Input: part model. Units: mm. Frame: model coordinates. A direction names the side the tool comes from. Give positions to 0.01 mm unless a question says otherwise; leave off trailing zeros. Loops run counter-clockwise (first coordinate to the right, second up) from the corner with the lowest first, then second, coordinate; pieces in that order, holes last. Notation, with made-up numbers: M 27,61.5 L 75,61.5 A10 cw 75,71.5 Z; hole C 10,-21 d10. An arc over 180 degrees is marked long. Use a Markdown table: item, result. Add a question column.
from build123d import *

# Parameters (mm, degrees)
CROQUIS1_W              = 45
CROQUIS1_H              = 20
SALIENTE_EXTRUIR1_DEPTH = 10
CROQUIS2_W              = 40.2
CROQUIS2_H              = 16.2
CORTAR_EXTRUIR1_DEPTH   = 8
CROQUIS3_W              = 14
CROQUIS3_H              = 7
CORTAR_EXTRUIR2_DEPTH   = 8
CROQUIS4_W              = 20
CROQUIS4_H              = 8
CORTAR_EXTRUIR3_DEPTH   = 8


with BuildPart() as part:
    # Croquis1 → Saliente-Extruir1 (new body)
    with BuildSketch(Plane(origin=(0, 0, 0), x_dir=(1, 0, 0), z_dir=(0, 1, 0))):
        Rectangle(CROQUIS1_W, CROQUIS1_H)
    extrude(amount=SALIENTE_EXTRUIR1_DEPTH)

    # Croquis2 → Cortar-Extruir1 (cut)
    with BuildSketch(Plane(origin=(0, 10, 0), x_dir=(1, 0, 0), z_dir=(0, 1, 0))):
        Rectangle(CROQUIS2_W, CROQUIS2_H)
    extrude(amount=-CORTAR_EXTRUIR1_DEPTH, mode=Mode.SUBTRACT)

    # Croquis3 → Cortar-Extruir2 (cut)
    with BuildSketch(Plane(origin=(22.5, 0, 0), x_dir=(0, 0, -1), z_dir=(1, 0, 0))):
        with Locations((0, 6.5)):
            Rectangle(CROQUIS3_W, CROQUIS3_H)
    extrude(amount=-CORTAR_EXTRUIR2_DEPTH, mode=Mode.SUBTRACT)

    # Croquis4 → Cortar-Extruir3 (cut)
    with BuildSketch(Plane.XY.offset(10)):
        with Locations((-10.1, 6)):
            Rectangle(CROQUIS4_W, CROQUIS4_H)
    extrude(amount=-CORTAR_EXTRUIR3_DEPTH, mode=Mode.SUBTRACT)


solid = part.part
1) Reachability of faces 5 (the flat face through (21, 6, 7)), 6 (the flat face through (-22.5, 5, 0)), 7 (the flat face through (0, 6, -8.1)), 8 (the flat face through (-0.1, 6, 9)) from +Z, -Z, +X, -X, +Y, -Y: full face, straight path, thin tool, end or side. Return the list, or none.
2) Ray query, line 1 (Z direction, x = 18, y = 6.5); line 2 (X direction, y = 2.5, z = -0.5); line 3 (X direction, y = 9.75, z = 2.5). Return the intervals inside material, ascending. Write a range as [from, to].
3) Pull-direction query (X, two-part tool) for faces 1 (the flat face through (22.5, 2.7, 0.1)), 2 (the flat face through (0, 2, 1)), 3 (the flat face through (10, 6, 8.1)), 4 (the flat face through (21, 6, -7)); classes: pulls with the +X half, pulls with the -X half, needs draft (parallel to the pull), parting line crosses it, or undercut.
4) Contact query for flat-ended pins moving along their axis: P1, Ø5, axis at x = -1, z = -2.5, coming from the +Y side; P2, Ø1.9, axis at x = 21.5, z = -3, coming from the +Y side; P3, Ø2.5, axis at y = 5, z = 2, coming from the +X side. Output: stop coordinate, or through.
5) Section query B-B, the plane z = -3. Return the cut outline in (x, y).
6) Section query C-C, the plane x = 17.5. Return the cut outline in (y, z), and give its area (3 significant figures).
7) Section query A-A, the plane y = 5.5. Return the cut outline in (x, z).
Entries:
| question | item | result |
|---|---|---|
| 1 | face 5 | +X, +Y |
| 1 | face 6 | +Z, -Z, -X, +Y, -Y |
| 1 | face 7 | +Y |
| 1 | face 8 | +Z, +Y |
| 2 | line 1 | z = [-10, -8.1], [8.1, 10] |
| 2 | line 2 | x = [-22.5, -20.1], [20.1, 22.5] |
| 2 | line 3 | x = [-22.5, -20.1] |
| 3 | face 1 | pulls with the +X half |
| 3 | face 2 | undercut |
| 3 | face 3 | undercut |
| 3 | face 4 | needs draft |
| 4 | P1 | stops at y = 2 |
| 4 | P2 | stops at y = 3 |
| 4 | P3 | stops at x = -20.1 |
| 5 | outline | M -22.5,0 L 22.5,0 L 22.5,3 L 20.1,3 L 20.1,2 L -20.1,2 L -20.1,10 L -22.5,10 Z |
| 6 | outline | M 0,-10 L 10,-10 L 10,-8.1 L 2,-8.1 L 2,8.1 L 10,8.1 L 10,10 L 0,10 Z |
| 6 | area | 70.4 mm² |
| 7 | outline | M -22.5,-10 L 22.5,-10 L 22.5,-7 L 20.1,-7 L 20.1,-8.1 L -20.1,-8.1 L -20.1,10 L -22.5,10 Z; M -0.1,8.1 L 20.1,8.1 L 20.1,7 L 22.5,7 L 22.5,10 L -0.1,10 Z |
